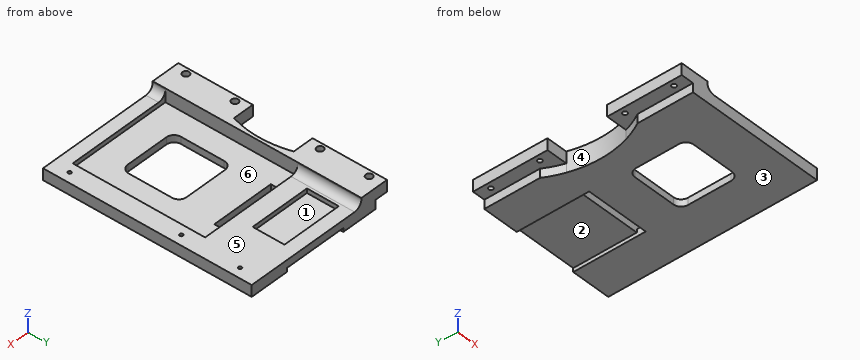
Autodesk Inventor part; units mm, degrees
ref_plane "YZ Plane" through (0, 0, 0) normal (1, 0, 0) x (0, 1, 0)
ref_plane "XZ Plane" through (0, 0, 0) normal (0, 1, 0) x (-1, 0, 0)
ref_plane "XY Plane" through (0, 0, 0) normal (0, 0, 1) x (1, 0, 0)
sketch "Sketch1" plane through (0, 0, 0) normal (0, 0, 1) x (1, 0, 0)
  line L0 (0, 0) -> (0, 22.958) construction
  line L1 (0, 0) -> (0, -22.958) construction
  line L2 (0, -22.958) -> (16.63, -22.958) construction
  line L3 (16.63, -22.958) -> (16.63, -81.958) construction
  line L4 (16.63, -81.958) -> (0, -81.958) construction
  line L5 (0, -81.958) -> (0, -22.958) construction
  line L6 (0, 22.958) -> (16.63, 22.958) construction
  line L7 (16.63, 22.958) -> (16.63, 81.958) construction
  line L8 (16.63, 81.958) -> (0, 81.958) construction
  line L9 (0, 81.958) -> (0, 22.958) construction
  line L10 (0, -52.458) -> (0.5, -52.458) construction
  line L11 (8.315, -22.958) -> (8.315, -23.458) construction
  line L12 (0, 0) -> (-53.686, 0) construction
  circle A0 centre (-53.686, 0) radius 74 construction
  line L13 (20.314, 0) -> (20.814, 0) construction
  line L14 (16.63, -22.958) -> (17.13, -22.958) construction
  line L15 (16.63, 22.958) -> (17.13, 22.958) construction
  line L16 (0.5, -23.458) -> (17.13, -23.458)
  line L17 (17.13, -23.458) -> (17.13, -81.958)
  line L18 (17.13, -81.958) -> (0.5, -81.958)
  line L19 (0.5, -81.958) -> (0.5, -23.458)
  line L20 (8.315, 22.958) -> (8.315, 23.458) construction
  line L21 (0.5, 81.958) -> (17.13, 81.958)
  line L22 (17.13, 81.958) -> (17.13, 23.458)
  line L23 (17.13, 23.458) -> (0.5, 23.458)
  line L24 (0.5, 23.458) -> (0.5, 81.958)
  arc A1 (17.13, -23.458) -> (17.13, 23.458) centre (-55.7128, 0) ccw
  line L25 (17.13, -81.958) -> (23.13, -81.958)
  line L26 (23.13, -81.958) -> (23.13, 81.958)
  line L27 (23.13, 81.958) -> (17.13, 81.958)
  dimension "d8" = 148
  dimension "d0" = 22.958
  dimension "d1" = 22.958
  dimension "d2" = 16.63
  dimension "d3" = 59
  dimension "d5" = 0.5
  dimension "d6" = 0.5
  dimension "d7" = 53.686
  dimension "d9" = 0.5
  dimension "d10" = 0.5
  dimension "d11" = 0.5
  dimension "d13" = 0.5
  dimension "d14" = 6
extrude "Extrusion1" add sketch "Sketch1" along normal blind 9
sketch "Sketch2" plane through (0, 0, 0) normal (0, 0, -1) x (-1, 0, 0)
  line L0 (-16.63, 22.958) -> (-16.63, 81.958) construction
  circle A0 centre (53.686, 0) radius 74 construction
  line L1 (-16.63, -22.958) -> (-16.63, -81.958) construction
  line L2 (-0.5, 23.458) -> (-17.13, 23.458)
  line L3 (-16.63, 23.458) -> (-16.63, 81.958)
  line L4 (-23.13, 81.958) -> (-0.5, 81.958)
  line L5 (-17.13, -23.458) -> (-0.5, -23.458)
  line L6 (-16.63, -23.458) -> (-16.63, -81.958)
  line L7 (-0.5, -81.958) -> (-23.13, -81.958)
  arc A1 (-17.13, 23.458) -> (-17.13, -23.458) centre (55.7128, 0) ccw
  arc A2 (-17.13, 23.458) -> (-17.13, -23.458) centre (55.7128, 0) ccw
  line L8 (-23.13, 81.958) -> (-110.13, 81.958)
  line L9 (-110.13, 81.958) -> (-110.13, -81.958)
  line L10 (-110.13, -81.958) -> (-23.13, -81.958)
  line L11 (-23.13, -81.958) -> (-23.13, 81.958)
  line L12 (0, 0) -> (-10.5, 0) construction
  line L13 (-0.5, -81.958) -> (-23.13, -81.958)
  arc A3 (-10.5, 38.3695) -> (-10.5, -38.3695) centre (55.7128, 0) ccw
  line L14 (-10.5, 38.3695) -> (-10.5, 81.958)
  line L15 (-10.5, -38.3695) -> (-10.5, -81.958)
  point P0 (-10, 81.958)
  dimension "d17" = 87
  dimension "d66" = 10.5
extrude "Extrusion2" add sketch "Sketch2" along normal blind 7 and the other way blind 2 contours A1 A3 L6 L7 L11 L4 L3 | L3 L4 L14 A3 | A3 L15 L7 L6 | L11 L10 L9 L8
sketch "Sketch3" plane through (0, 0, 9) normal (0, 0, 1) x (1, 0, 0)
  line L0 (0.5, -81.958) -> (23.13, -81.958) construction
  line L1 (0, -23.458) -> (10, -23.458) construction
  line L2 (10, -23.458) -> (10, -81.958) construction
  line L3 (10, -81.958) -> (0, -81.958) construction
  line L4 (0, -81.958) -> (0, -23.458) construction
  line L5 (0, 23.458) -> (10, 23.458) construction
  line L6 (0, 81.958) -> (0, 23.458) construction
  line L7 (5, -81.958) -> (5, -71.958) construction
  line L8 (17.13, -23.458) -> (0.5, -23.458) construction
  line L9 (5, -23.458) -> (5, -33.458) construction
  line L10 (5, -23.458) -> (15, -23.458) construction
  circle A0 centre (5, -71.958) radius 1.75
  circle A1 centre (5, -33.458) radius 1.75
  line L11 (-21.548, 0) -> (41.2165, 0) construction
  circle A2 centre (5, 71.958) radius 1.75
  circle A3 centre (5, 33.458) radius 1.75
  point P0 (0, 0)
  dimension "d20" = 10
  dimension "d21" = 10
  dimension "d22" = 10
  dimension "d24" = 3.5
  dimension "d25" = 3.5
extrude "Extrusion3" cut sketch "Sketch3" against normal up to surface (9 mm away)
sketch "Sketch4" plane through (0, 0, 9) normal (0, 0, 1) x (1, 0, 0)
  circle A0 centre (5, -71.958) radius 1.75
  circle A1 centre (5, -71.958) radius 2.65
  circle A2 centre (5, -33.458) radius 1.75
  circle A3 centre (5, -33.458) radius 2.65
  circle A4 centre (5, 33.458) radius 1.75
  circle A5 centre (5, 33.458) radius 2.65
  circle A6 centre (5, 71.958) radius 1.75
  circle A7 centre (5, 71.958) radius 2.65
  point P0 (0, 0)
  dimension "d28" = 5.3
  dimension "d29" = 5.3
extrude "Extrusion4" cut sketch "Sketch4" against normal blind 6 contours A0 | A1 | A2 | A3 | A4 | A5 | A6 | A7
sketch "Sketch5" plane through (0, 0, 2) normal (0, 0, 1) x (1, 0, 0)
  line L0 (23.13, -71.958) -> (105.13, -71.958)
  line L1 (105.13, -71.958) -> (105.13, 32.042)
  line L2 (105.13, 32.042) -> (23.13, 32.042)
  line L3 (23.13, 32.042) -> (23.13, -71.958)
  line L4 (31.2383, 46.3792) -> (79.2383, 46.3792)
  line L5 (79.2383, 46.3792) -> (79.2383, 71.3792)
  line L6 (79.2383, 71.3792) -> (31.2383, 71.3792)
  line L7 (31.2383, 71.3792) -> (31.2383, 46.3792)
  line L8 (23.13, -81.958) -> (23.13, 81.958) construction
  line L9 (23.13, -81.958) -> (23.13, 81.958) construction
  line L10 (23.13, -81.958) -> (23.13, -71.958) construction
  point P0 (0, 0)
  dimension "d34" = 82
  dimension "d35" = 104
  dimension "d36" = 48
  dimension "d37" = 25
  dimension "d38" = 10
extrude "Extrusion5" cut sketch "Sketch5" against normal blind 3.5
sketch "Sketch6" plane through (0, 0, 2) normal (0, 0, 1) x (1, 0, 0)
  line L0 (23.13, 32.042) -> (105.13, 32.042)
  line L1 (64.13, 32.042) -> (39.13, 32.042)
  line L2 (64.13, 32.042) -> (89.13, 32.042)
  line L3 (89.13, 32.042) -> (89.13, 25.042)
  line L4 (89.13, 25.042) -> (39.13, 25.042)
  line L5 (39.13, 25.042) -> (39.13, 32.042)
  point P0 (0, 0)
  dimension "d41" = 25
  dimension "d42" = 25
  dimension "d43" = 7
extrude "Extrusion6" cut sketch "Sketch6" against normal up to surface (9 mm away)
sketch "Sketch7" plane through (23.13, 32.042, 2) normal (0, -1, 0) x (1, 0, 0)
  line L0 (66, -9) -> (16, -9)
  line L1 (66, -3.5) -> (66, -9)
  line L2 (16, -9) -> (66, -9)
  line L3 (66, -9) -> (66, -6)
  line L4 (66, -6) -> (16, -6)
  line L5 (16, -6) -> (16, -9)
  point P0 (-23.13, -2)
  dimension "d46" = 3
extrude "Extrusion7" cut sketch "Sketch7" against normal up to surface (49.916 mm away)
sketch "Sketch8" plane through (0, 0, -1.5) normal (0, 0, 1) x (1, 0, 0)
  line L0 (41.13, -49.8888) -> (87.13, -49.8888)
  line L1 (87.13, -49.8888) -> (87.13, -3.8888)
  line L2 (87.13, -3.8888) -> (41.13, -3.8888)
  line L3 (41.13, -3.8888) -> (41.13, -49.8888)
  line L4 (41.13, -49.8888) -> (87.13, -3.8888) construction
  line L5 (87.13, -49.8888) -> (41.13, -3.8888) construction
  point P0 (0, 0)
  point P1 (64.13, -26.8888)
  dimension "d49" = 46
  dimension "d50" = 46
extrude "Extrusion8" cut sketch "Sketch8" against normal up to surface (5.5 mm away)
sketch "Sketch9" plane through (0, 0, 2) normal (0, 0, 1) x (1, 0, 0)
  line L0 (110.13, 81.958) -> (110.13, -81.958)
  line L1 (110.13, -81.958) -> (120.13, -81.958)
  line L2 (120.13, -81.958) -> (120.13, 81.958)
  line L3 (120.13, 81.958) -> (110.13, 81.958)
  line L4 (110.13, 81.958) -> (110.13, -81.958)
  point P0 (0, 0)
  dimension "d53" = 10
extrude "Extrusion9" add sketch "Sketch9" against normal blind 9
sketch "Sketch10" plane through (0, 0, 2) normal (0, 0, 1) x (1, 0, 0)
  line L0 (105.13, 32.042) -> (105.13, -71.958) construction
  line L1 (105.13, -71.958) -> (120.13, -71.958) construction
  line L2 (120.13, -81.958) -> (120.13, 81.958) construction
  circle A0 centre (112.63, -67.7077) radius 1.275
  circle A1 centre (112.63, 66.21) radius 1.275
  circle A2 centre (112.63, 20.0315) radius 1.275
  line L3 (23.13, -81.958) -> (120.13, -81.958) construction
  line L4 (112.63, 66.21) -> (112.63, 81.958) construction
  line L5 (89.13, 81.958) -> (120.13, 81.958) construction
  line L6 (112.63, 66.21) -> (112.63, 20.0315) construction
  line L7 (112.63, -67.7077) -> (112.63, -81.958) construction
  point P0 (0, 0)
  dimension "d56" = 2.55
  dimension "d57" = 2.55
  dimension "d58" = 2.55
  dimension "d60" = 15.748
  dimension "d61" = 46.1785
  dimension "d62" = 14.2503
extrude "Extrusion10" cut sketch "Sketch10" against normal blind 4.5
fillet "Fillet1" radius 6 6 edges at (41.13, -49.8888, -4.25) (41.13, -3.8888, -4.25) (87.13, -3.8888, -4.25) (87.13, -49.8888, -4.25) (23.13, -76.958, 2) (23.13, 57, 2)
properties part number "Base Extension 1"
Could you check a few things on this model? Use its own coordinates, in mm. Face numbers are marked on the shaded views. A direction names the side the tool comes from. Coordinates: 2 decimals unless noted, no trailing zeros. Write each loop counter-clockwise with the first axis right and the second up, starting at its lowest first coordinate (ties: lowest second). Pieces come first, ordered by that corner, then holes. Notation, with made-up numbers: (41, -4) -> (66, -4) arc R8 ccw to (66, 9) -> close; hole circle Ø3 at (-28, 43.5). An arc over 180 degrees is marked (long way). One line per question, with ' | ' between items. Start each with the question number.
1. If we section it at A-A (z = 6): Please give me the cut outline in (x, y), and give its area (3 significant figures).
2. For the marked faces 1, 2 and 3, which set-ups out of +Z, -Z, +X, -X, +Y, -Y let a thin tool reach every point of the face, with its end or its side?
3. If we section it at B-B (y = -6.5): Please give me the cut outline in (x, z).
4. Thinking about a two-plate mould opening in X: for the marked faces 4, 5 and 6, which applies, pulls with the +X half, pulls with the -X half, needs draft (parallel to the pull), parting line crosses it, or undercut?
5. If we section it at C-C (x = 5): Count the separate pieces of the cut face and the enclosed holes in it, and give its area (3 significant figures).
6. Please list where these lines run through material, in increasing order: line 1 along Y through (x, z) = (5, 5.85); line 2 along Y through (x, z) = (5, 1.9); line 3 along Y through (x, z) = (112.63, 1.15) (1 decimal).
7. Will these pins go through, and if not, where does the flat tip stop? P1, Ø2, axis at x = 78, y = 44, coming from the +Z side; P2, Ø4, axis at x = 5, y = -71.958, coming from the -Z side; P3, Ø1.5, axis at y = 13, z = 5.5, coming from the -X side.
Return value:
1) outline: (0.5, -81.96) -> (23.47, -81.96) -> (23.47, -71.96) -> (23.13, -71.96) -> (23.13, 32.04) -> (23.47, 32.04) -> (23.47, 81.96) -> (0.5, 81.96) -> (0.5, 23.46) -> (17.13, 23.46) arc R76.53 cw to (17.13, -23.46) -> (0.5, -23.46) -> close; hole circle Ø5.3 at (5, -71.96); hole circle Ø5.3 at (5, -33.46); hole circle Ø5.3 at (5, 33.46); hole circle Ø5.3 at (5, 71.96) | area: 2,750 mm²
2) face 1: +Z | face 2: -Z, +Y | face 3: -Z, +X, -X, +Y, -Y
3) outline: (20.54, -7) -> (42.18, -7) -> (42.18, -1.5) -> (23.13, -1.5) -> (23.13, 9) -> (20.54, 9) -> close; (86.08, -7) -> (120.13, -7) -> (120.13, 2) -> (105.13, 2) -> (105.13, -1.5) -> (86.08, -1.5) -> close
4) face 4: pulls with the -X half | face 5: needs draft | face 6: undercut
5) separate pieces: 6 | enclosed holes: 0 | area: 884 mm²
6) line 1: y = -81.96 to -74.61, -69.31 to -36.11, -30.81 to -23.46, 23.46 to 30.81, 36.11 to 69.31, 74.61 to 81.96 | line 2: y = -81.96 to -73.71, -70.21 to -35.21, -31.71 to -23.46, 23.46 to 31.71, 35.21 to 70.21, 73.71 to 81.96 | line 3: y = -82 to -69, -66.4 to 18.8, 21.3 to 64.9, 67.5 to 82
7) P1: stops at z = 2 | P2: stops at z = 0 | P3: stops at x = 19.57
